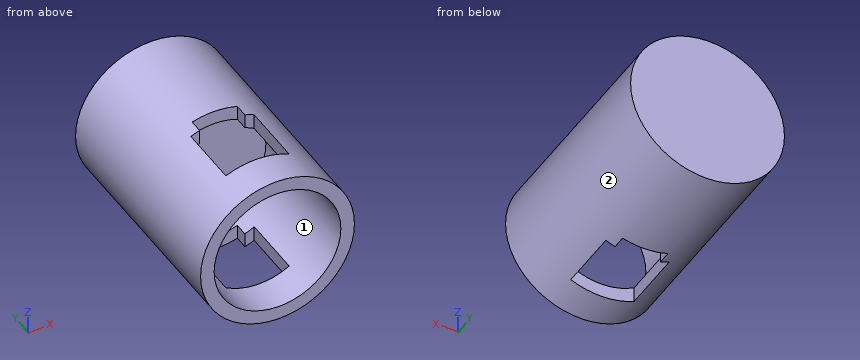
```python
from build123d import *

# Parameters (mm, degrees)
SKETCH1_R               = 17
BOSS_EXTRUDE1_DEPTH     = 30
SKETCH2_R               = 14
CUT_EXTRUDE1_DEPTH      = 30
SKETCH3_W               = 14
SKETCH3_H               = 14
CUT_EXTRUDE2_DEPTH      = 18
CUT_EXTRUDE2_DEPTH_BACK = 18
SKETCH4_R               = 17
BOSS_EXTRUDE2_DEPTH     = 20
SKETCH6_W               = 10
SKETCH6_H               = 6
CUT_EXTRUDE3_DEPTH      = 18
CUT_EXTRUDE3_DEPTH_BACK = 18


with BuildPart() as part:
    # Sketch1 → Boss-Extrude1 (new body)
    with BuildSketch(Plane(origin=(0, 0, 0), x_dir=(1, 0, 0), z_dir=(0, 1, 0))):
        Circle(SKETCH1_R)
    extrude(amount=BOSS_EXTRUDE1_DEPTH)

    # Sketch2 → Cut-Extrude1 (cut)
    with BuildSketch(Plane(origin=(0, 30, 0), x_dir=(1, 0, 0), z_dir=(0, 1, 0))):
        Circle(SKETCH2_R)
    extrude(amount=-CUT_EXTRUDE1_DEPTH, mode=Mode.SUBTRACT)

    # Sketch3 → Cut-Extrude2 (cut, two sides)
    with BuildSketch(Plane.XY) as cut_extrude2_sk:
        with Locations((0, 15)):
            Rectangle(SKETCH3_W, SKETCH3_H)
    extrude(amount=CUT_EXTRUDE2_DEPTH, mode=Mode.SUBTRACT)
    extrude(cut_extrude2_sk.sketch, amount=-CUT_EXTRUDE2_DEPTH_BACK, mode=Mode.SUBTRACT)

    # Sketch4 → Boss-Extrude2 (add)
    with BuildSketch(Plane(origin=(0, 30, 0), x_dir=(1, 0, 0), z_dir=(0, 1, 0))):
        Circle(SKETCH4_R)
    extrude(amount=BOSS_EXTRUDE2_DEPTH)

    # Sketch6 → Cut-Extrude3 (cut, two sides)
    with BuildSketch(Plane.XY) as cut_extrude3_sk:
        with Locations((-0.049003827, 22)):
            Rectangle(SKETCH6_W, SKETCH6_H)
    extrude(amount=CUT_EXTRUDE3_DEPTH, mode=Mode.SUBTRACT)
    extrude(cut_extrude3_sk.sketch, amount=-CUT_EXTRUDE3_DEPTH_BACK, mode=Mode.SUBTRACT)


solid = part.part
```
Verification items for the finished model (mm, model axes). Face numbers are marked on the shaded views. A direction names the side the tool comes from. Round coordinates to 2 decimals unless told otherwise and drop trailing zeros. Write each loop counter-clockwise with the first axis right and the second up, starting at its lowest first coordinate (ties: lowest second). Pieces come first, ordered by that corner, then holes. Notation, with made-up numbers: (68, 13.5) - (112, 13.5) arc R4 cw to (112, 18.5) - close; hole circle Ø3 at (53, 15.5). An arc over 180 degrees is marked (long way). Answer as a JSON object with one key per item and string values. Group by question number.
Q1. Go/stop test with flat-tipped pins: pin 1 Ø4 at (x, y) = (12, 5.5) entering from -Z; pin 2 Ø2.5 at (y, z) = (16.5, -13.5) entering from -X; pin 3 Ø1 at (y, z) = (16.5, 13) entering from -X. Record where each tip stops, or that it passes through.
Q2. Section check A-A, the plane y = 17.5. Enter the section's corners in (x, z).
Q3. Thickness scan on line 1 (X direction, y = 10, z = 0); line 2 (Y direction, x = -7, z = 4); line 3 (Z direction, x = 7, y = 4). Record the ranges inside material, lowest first.
Q4. Section check D-D, the plane x = 0. Enter the section's corners in (y, z), plus the area to 3 significant figures.
Q5. Section check C-C, the plane z = 0. Enter the section's corners in (x, y), plus the area to 3 significant figures.
Q6. Tool access check on the marked faces 1 and 2. Record the directions out of +Z, -Z, +X, -X, +Y, -Y that give a thin tool (end or side, any length) a straight path to the whole face; none if there is none.
Q7. Section check B-B, the plane x = 4. Enter the section's corners in (y, z), plus the area to 3 significant figures.
Found:
{
 "1": {"pin 1": "stops at z = -13.75", "pin 2": "stops at x = -11.79", "pin 3": "stops at x = -11.52"},
 "2": {"outline": "(-7, -15.49) - (-7, -12.12) arc R14 cw to (-7, 12.12) - (-7, 15.49) arc R17 ccw to start; (7, -15.49) arc R17 ccw to (7, 15.49) - (7, 12.12) arc R14 cw to (7, -12.12) - close"},
 "3": {"line 1": "x = -17 to -14, 14 to 17", "line 2": "y = 30 to 50", "line 3": "z = -15.49 to -12.12, 12.12 to 15.49"},
 "4": {"outline": "(0, -17) - (8, -17) - (8, -14) - (0, -14) - close; (0, 14) - (8, 14) - (8, 17) - (0, 17) - close; (25, -17) - (50, -17) - (50, 17) - (25, 17) - (25, 14) - (30, 14) - (30, -14) - (25, -14) - close", "area": "758 mm^2"},
 "5": {"outline": "(-17, 0) - (-14, 0) - (-14, 30) - (14, 30) - (14, 0) - (17, 0) - (17, 50) - (-17, 50) - close", "area": "860 mm^2"},
 "6": {"face 1": "-Y", "face 2": "+Y, -Y"},
 "7": {"outline": "(0, -16.52) - (8, -16.52) - (8, -13.42) - (0, -13.42) - close; (0, 13.42) - (8, 13.42) - (8, 16.52) - (0, 16.52) - close; (25, -16.52) - (50, -16.52) - (50, 16.52) - (25, 16.52) - (25, 13.42) - (30, 13.42) - (30, -13.42) - (25, -13.42) - close", "area": "742 mm^2"}
}
